Here's how the part is built. I have some questions about the finished solid (model axes, mm). A direction names the side the tool comes from. Give positions to 0.01 mm unless a question says otherwise; leave off trailing zeros. Loops run counter-clockwise (first coordinate to the right, second up) from the corner with the lowest first, then second, coordinate; pieces in that order, holes last.
Q1. If we section it at D-D (z = 12.5): Please give me the cut outline in (x, y).
Q2. Will these pins go through, and if not, where does the flat tip stop? P1, Ø10, axis at y = -12.5, z = 28, coming from the -X side; P2, Ø21.5, axis at x = 34.5, z = 22, coming from the -Y side; P3, Ø8, axis at x = 53.5, z = 24, coming from the +Y side; P4, Ø8, axis at y = -11.5, z = 39, coming from the +X side.
Q3. We'd pull the mould along Y, two halves only. Please class faces 1 (the face through (53.03, -9.42, 28.75)), 2 (the face through (42.04, 3.8, 45.81)), 3 (the face through (59.55, 11.046, 4.521)): +Y half, -Y half, draft (parallel to the pull), parting line (faces both ways), or undercut.
Q4. If we section it at B-B (y = 5): Please give me the cut outline in (x, z).
Q5. I need wall thicknesses on line 1 (Y direction, x = 61, z = 2); line 2 (X direction, y = 14.5, z = 15); line 3 (X direction, y = 4, z = 12). Which ranges of each line are inside material? Lowest first, please.
Q6. If we section it at A-A (z = 23.5): Please give me the cut outline in (x, y), plus the area to 3 significant figures.
Q7. If we section it at C-C (x = 27.5): Please give me the cut outline in (y, z), plus the area to 3 significant figures.
Q8. For faces 4 (the face through (-6, 16, 3)), 5 (the face through (-8, -15, 3)), 6 (the face through (15.94, 3.8, 37.02)), 7 (the face through (51, 11, 18)), 8 (the face through (55, 1, 22)), which set-ups out of +Z, -Z, +X, -X, +Y, -Y let a thin tool reach every point of the face, with its end or its side?
from build123d import *

# Parameters (mm, degrees)
BOSS_EXTRUDE1_DEPTH  = 49
SKETCH2_R            = 2.5
CUT_EXTRUDE1_DEPTH   = 8.5
SKETCH4_W            = 79
SKETCH4_H            = 39.5
BOSS_EXTRUDE2_DEPTH  = 6
BOSS_EXTRUDE3_DEPTH  = 4
SKETCH5_R            = 2
CUT_EXTRUDE3_DEPTH   = 10
BOSS_EXTRUDE4_DEPTH  = 4
FILLET1_R            = 6
FILLET2_R            = 5
CUT_EXTRUDE5_DEPTH   = 3
CUT_EXTRUDE6_DEPTH   = 50
CUT_EXTRUDE7_DEPTH   = 3
LPATTERN1_COUNT      = 2
LPATTERN1_PITCH      = 67
LPATTERN1_COUNT_DIR2 = 2
LPATTERN1_PITCH_DIR2 = 27.5
BOSS_EXTRUDE5_DEPTH  = 10


with BuildPart() as part:
    # Sketch1 → Boss-Extrude1 (new body)
    with BuildSketch(Plane.XY):
        Polygon((4, 7.5), (4, 19.5), (0, 19.5), (0, 0), (55, 0), (55, 7.5), align=None)
    extrude(amount=BOSS_EXTRUDE1_DEPTH)

    # Sketch2 → Cut-Extrude1 (cut, through all)
    with BuildSketch(Plane(origin=(0, 7.5, 0), x_dir=(1, 0, 0), z_dir=(0, 1, 0))):
        with Locations(Location((12, -12.5, 0), (0, 0, 270))):  # turned: the seam where the file's is
            Circle(SKETCH2_R)
        with Locations(Location((43, -12.5, 0), (0, 0, 270))):  # turned: the seam where the file's is
            Circle(SKETCH2_R)
        with Locations(Location((12, -43.5, 0), (0, 0, 270))):  # turned: the seam where the file's is
            Circle(SKETCH2_R)
        with Locations(Location((43, -43.5, 0), (0, 0, 270))):  # turned: the seam where the file's is
            Circle(SKETCH2_R)
        with BuildLine():
            Line((14.460001345, -31.494057109), (19.150704606, -49))
            Line((19.150704606, -49), (35.849295394, -49))
            Line((35.849295394, -49), (40.539998655, -31.494057109))
            ThreePointArc((40.539998655, -31.494057109), (27.5, -14.5), (14.460001345, -31.494057109))
        make_face()
    extrude(amount=-CUT_EXTRUDE1_DEPTH, mode=Mode.SUBTRACT)

    # Sketch4 → Boss-Extrude2 (add)
    with BuildSketch(Plane(origin=(0, 0, 0), x_dir=(-1, 0, 0), z_dir=(0, 0, -1))):
        with Locations((-27.5, -0.25)):
            Rectangle(SKETCH4_W, SKETCH4_H)
    extrude(amount=-BOSS_EXTRUDE2_DEPTH)

    # Sketch6 → Boss-Extrude3 (add)
    with BuildSketch(Plane.ZY):
        Polygon((6, -20), (49, 0), (6, 0), align=None)
    extrude(amount=-BOSS_EXTRUDE3_DEPTH)

    # Sketch5 → Cut-Extrude3 (cut)
    with BuildSketch(Plane(origin=(0, 0, 0), x_dir=(-1, 0, 0), z_dir=(0, 0, -1))):
        with Locations((-61, 13.5)):
            Circle(SKETCH5_R)
        with Locations((-61, -14)):
            Circle(SKETCH5_R)
        with Locations((6, 13.5)):
            Circle(SKETCH5_R)
        with Locations((6, -14)):
            Circle(SKETCH5_R)
    extrude(amount=-CUT_EXTRUDE3_DEPTH, mode=Mode.SUBTRACT)

    # Sketch7 → Boss-Extrude4 (add)
    with BuildSketch(Plane(origin=(55, 0, 0), x_dir=(0, 0, -1), z_dir=(1, 0, 0))):
        Polygon((-49, 7.5), (-6, 19.5), (0, 19.5), (0, -20), (-6, -20), (-49, 0), align=None)
    extrude(amount=-BOSS_EXTRUDE4_DEPTH)

    # Fillet1
    fillet1_edges = [part.edges().sort_by_distance(p)[0] for p in [
        (67, 19.5, 3),
        (-12, 19.5, 3),
        (-12, -20, 3),
        (67, -20, 3),
    ]]
    fillet(fillet1_edges, radius=FILLET1_R)

    # Fillet2
    fillet2_edges = [part.edges().sort_by_distance(p)[0] for p in [
        (35.849295394, 3.75, 49),
        (19.150704606, 3.75, 49),
    ]]
    fillet(fillet2_edges, radius=FILLET2_R)

    # Sketch9 → Cut-Extrude5 (cut)
    with BuildSketch(Plane.XY.offset(6)):
        Polygon((-6, 16.790896534), (-8.85, 15.145448267), (-8.85, 11.854551733), (-6, 10.209103466), (-3.15, 11.854551733), (-3.15, 15.145448267), align=None)
        Polygon((-6, -10.709103466), (-8.85, -12.354551733), (-8.85, -15.645448267), (-6, -17.290896534), (-3.15, -15.645448267), (-3.15, -12.354551733), align=None)
        Polygon((61, -10.709103466), (58.15, -12.354551733), (58.15, -15.645448267), (61, -17.290896534), (63.85, -15.645448267), (63.85, -12.354551733), align=None)
        Polygon((61, 10.209103466), (63.85, 11.854551733), (63.85, 15.145448267), (61, 16.790896534), (58.15, 15.145448267), (58.15, 11.854551733), align=None)
    extrude(amount=-CUT_EXTRUDE5_DEPTH, mode=Mode.SUBTRACT)

    # Sketch10 → Cut-Extrude6 (cut, through all)
    with BuildSketch(Plane(origin=(0, 0, 0), x_dir=(-1, 0, 0), z_dir=(0, 0, -1))):
        with BuildLine():
            Line((-61, 19.5), (-61, 26.194717678))
            Line((-61, 26.194717678), (-93.21372943, 26.194717678))
            Line((-93.21372943, 26.194717678), (-93.21372943, -32.483465835))
            Line((-93.21372943, -32.483465835), (20.656804912, -32.483465835))
            Line((20.656804912, -32.483465835), (20.656804912, 27.240467483))
            Line((20.656804912, 27.240467483), (6, 27.240467483))
            Line((6, 27.240467483), (6, 19.5))
            ThreePointArc((6, 19.5), (10.987484336, 16.835416016), (11.545111711, 11.208333333))
            ThreePointArc((11.545111711, 11.208333333), (9.270670267, -0.25), (11.545111711, -11.708333333))
            ThreePointArc((11.545111711, -11.708333333), (10.460015748, -18.013509627), (4.303797468, -19.755249514))
            ThreePointArc((4.303797468, -19.755249514), (-27.5, -15.166177907), (-59.303797468, -19.755249514))
            ThreePointArc((-59.303797468, -19.755249514), (-65.460015748, -18.013509627), (-66.545111711, -11.708333333))
            ThreePointArc((-66.545111711, -11.708333333), (-64.270670267, -0.25), (-66.545111711, 11.208333333))
            ThreePointArc((-66.545111711, 11.208333333), (-65.987484336, 16.835416016), (-61, 19.5))
        make_face()
    extrude(amount=-CUT_EXTRUDE6_DEPTH, mode=Mode.SUBTRACT)

    # Sketch11 → Cut-Extrude7 (cut)
    with BuildSketch(Plane.XY.offset(6)):
        with BuildLine():
            ThreePointArc((-9.35, 15.434123402), (-8.85, 13.5), (-9.35, 11.565876598))
            ThreePointArc((-9.35, 11.565876598), (-7.425, 11.031827599), (-6, 9.631753196))
            ThreePointArc((-6, 9.631753196), (-4.575, 11.031827599), (-2.65, 11.565876598))
            ThreePointArc((-2.65, 11.565876598), (-3.15, 13.5), (-2.65, 15.434123402))
            ThreePointArc((-2.65, 15.434123402), (-4.575, 15.968172401), (-6, 17.368246804))
            ThreePointArc((-6, 17.368246804), (-7.425, 15.968172401), (-9.35, 15.434123402))
        make_face()
    cut_extrude7 = extrude(amount=-CUT_EXTRUDE7_DEPTH, mode=Mode.SUBTRACT)

    # LPattern1: Cut-Extrude7 2 × 2
    with Locations(*[(i * LPATTERN1_PITCH, -j * LPATTERN1_PITCH_DIR2, 0) for i in range(LPATTERN1_COUNT) for j in range(LPATTERN1_COUNT_DIR2) if (i, j) != (0, 0)]):
        add(cut_extrude7, mode=Mode.SUBTRACT)

    # Sketch12 → Boss-Extrude5 (add)
    with BuildSketch(Plane(origin=(0, 19.5, 0), x_dir=(1, 0, 0), z_dir=(0, 1, 0))):
        Polygon((0, -49), (-6, -49), (-6, -45), (0, -28.515135483), align=None)
    extrude(amount=-BOSS_EXTRUDE5_DEPTH)


solid = part.part
Check sheet entries:
1. outline: (0, -16.98) - (4, -16.98) - (4, 0) - (9.5, 0) - (9.5, 7.5) - (4, 7.5) - (4, 19.5) - (0, 19.5) - close; (14.5, 0) - (40.5, 0) - (40.5, 7.5) - (14.5, 7.5) - close; (45.5, 0) - (51, 0) - (51, -16.98) - (55, -16.98) - (55, 17.69) - (51, 17.69) - (51, 7.5) - (45.5, 7.5) - close
2. P1: stops at x = 0
2. P2: stops at y = 0
2. P3: stops at y = 15.59
2. P4: passes through
3. face 1: -Y half
3. face 2: draft
3. face 3: undercut
4. outline: (-9.73, 0) - (64.73, 0) - (64.73, 6) - (55, 6) - (55, 49) - (42.37, 49) arc R5 ccw to (37.54, 42.71) - (40.54, 31.49) arc R13.5 cw (long way) to (14.46, 31.49) - (17.46, 42.71) arc R5 ccw to (12.63, 49) - (0, 49) - (0, 6) - (-9.73, 6) - close; hole circle Ø5 at (12, 12.5); hole circle Ø5 at (12, 43.5); hole circle Ø5 at (43, 12.5); hole circle Ø5 at (43, 43.5)
5. line 1: y = -20 to -16, -12 to 11.5, 15.5 to 19.5
5. line 2: x = 0 to 4, 51 to 55
5. line 3: x = 0 to 9.55, 14.45 to 40.55, 45.45 to 55
6. outline: (0, -11.86) - (4, -11.86) - (4, 0) - (14.77, 0) - (14.77, 7.5) - (4, 7.5) - (4, 19.5) - (0, 19.5) - close; (40.23, 0) - (51, 0) - (51, -11.86) - (55, -11.86) - (55, 14.62) - (51, 14.62) - (51, 7.5) - (40.23, 7.5) - close
6. area: 393 mm2
7. outline: (-15.17, 0) - (19.5, 0) - (19.5, 6) - (7.5, 6) - (7.5, 14.5) - (0, 14.5) - (0, 6) - (-15.17, 6) - close
7. area: 272 mm2
8. face 4: none
8. face 5: +Z
8. face 6: +Y, -Y
8. face 7: +Z, +Y
8. face 8: +Z, +X, +Y, -Y
